Geometry: see drawing. Coordinates: mm, zero at the bounding-box minimum. A direction names the side the tool comes from. Coordinates: 2 decimals unless noted, no trailing zeros. Order: outer loops, then holes, each group sorted by start corner. A loop starts at its lowest first (then second) coordinate and runs counter-clockwise, first axis right, second up. Notation, with made-up numbers: (24.5, -23) - (48.5, -23) arc R9 ccw to (48.5, -10) - close; hole circle Ø6 at (62.25, 18). An arc over 180 degrees is marked (long way). Use a Markdown table: item, result. Add a question column.
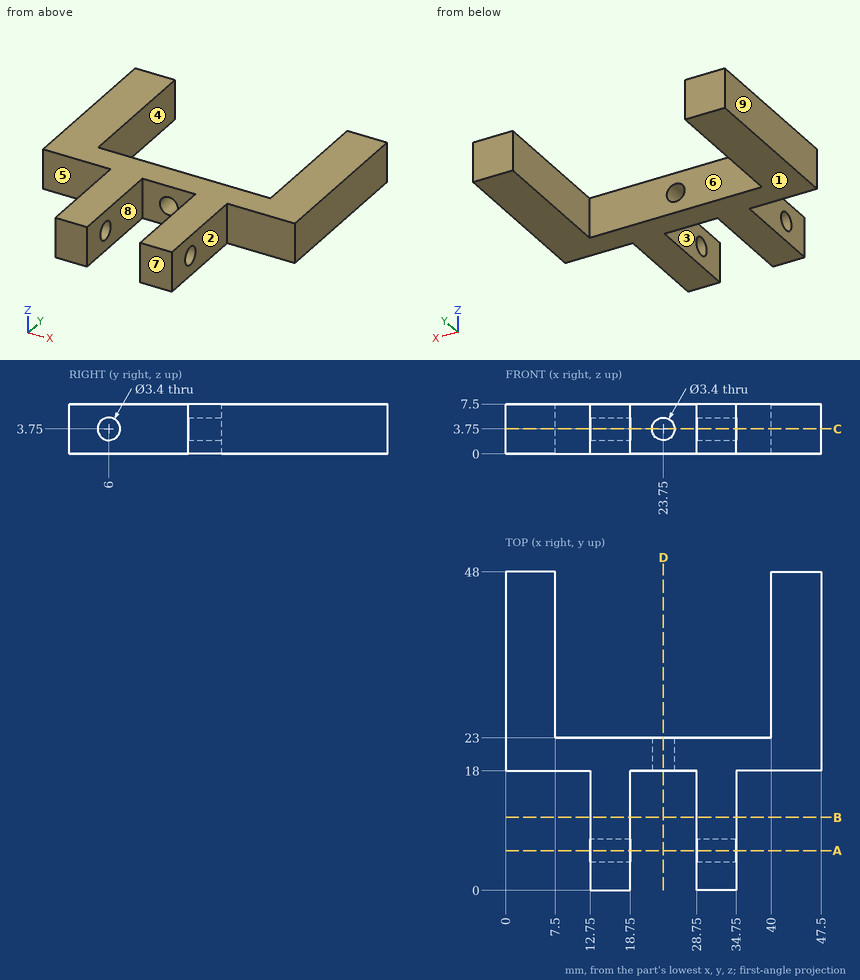
1) Section query B-B (y = 11). Return the cut outline in (x, z), and give its area (3 significant figures).
2) First-contact query: pin 1 (2 mm diameter, centred on y = 10, z = 2, fed in from +X); pin 2 (3 mm diameter, centred on x = 24.5, z = 5, fed in from -Y); pin 3 (1 mm diameter, centred on x = 25.5, z = 2, fed in from +Y); pin 4 (5 mm diameter, centred on x = 25, y = 27, fed in from -Z). Flat tips, straight axial feed; report the tip coordinate or a pass-through.
3) Line query: line 1 (X direction, y = 26, z = 4.5); line 2 (Z direction, x = 31.55, y = 6); line 3 (X direction, y = 14, z = 4.5). Output: solid intervals per line, ascending. Write a range as from..to.
4) Section query C-C (z = 3.75). Return the cut outline in (x, y).
5) Draft query along X for the marked faces 6, 7, 8 and 9. Return one class per face: released by +X, released by -X, zero draft, split by the parting line, or undercut.
6) Section query A-A (y = 6). Return the cut outline in (x, z).
7) Section query D-D (x = 23.75). Return the cut outline in (y, z), and give its area (3 significant figures).
8) Access query for the marked faces 1, 2, 3, 4 and 5. Directions: +Z, -Z, +X, -X, +Y, -Y. A direction counts if a zero-diameter tool reaches every point of the face in a straight line with its end or side. Return the directions, or none.
From the geometry:
| question | item | result |
|---|---|---|
| 1 | outline | (12.75, 0) - (18.75, 0) - (18.75, 7.5) - (12.75, 7.5) - close; (28.75, 0) - (34.75, 0) - (34.75, 7.5) - (28.75, 7.5) - close |
| 1 | area | 90.0 mm^2 |
| 2 | pin 1 | stops at x = 34.75 |
| 2 | pin 2 | stops at y = 18 |
| 2 | pin 3 | stops at y = 23 |
| 2 | pin 4 | passes through |
| 3 | line 1 | x = 0..7.5, 40..47.5 |
| 3 | line 2 | z = 0..2.05, 5.45..7.5 |
| 3 | line 3 | x = 12.75..18.75, 28.75..34.75 |
| 4 | outline | (0, 18) - (12.75, 18) - (12.75, 7.7) - (18.75, 7.7) - (18.75, 18) - (22.05, 18) - (22.05, 23) - (7.5, 23) - (7.5, 48) - (0, 48) - close; (12.75, 0) - (18.75, 0) - (18.75, 4.3) - (12.75, 4.3) - close; (25.45, 18) - (28.75, 18) - (28.75, 7.7) - (34.75, 7.7) - (34.75, 18) - (47.5, 18) - (47.5, 48) - (40, 48) - (40, 23) - (25.45, 23) - close; (28.75, 0) - (34.75, 0) - (34.75, 4.3) - (28.75, 4.3) - close |
| 5 | face 6 | undercut |
| 5 | face 7 | zero draft |
| 5 | face 8 | undercut |
| 5 | face 9 | released by -X |
| 6 | outline | (12.75, 0) - (18.75, 0) - (18.75, 2.05) - (12.75, 2.05) - close; (12.75, 5.45) - (18.75, 5.45) - (18.75, 7.5) - (12.75, 7.5) - close; (28.75, 0) - (34.75, 0) - (34.75, 2.05) - (28.75, 2.05) - close; (28.75, 5.45) - (34.75, 5.45) - (34.75, 7.5) - (28.75, 7.5) - close |
| 7 | outline | (18, 0) - (23, 0) - (23, 2.05) - (18, 2.05) - close; (18, 5.45) - (23, 5.45) - (23, 7.5) - (18, 7.5) - close |
| 7 | area | 20.5 mm^2 |
| 8 | face 1 | -Z, +X, -X, +Y, -Y |
| 8 | face 2 | +Z, -Z, +X, -Y |
| 8 | face 3 | +Z, -Z, -Y |
| 8 | face 4 | +Z, -Z, +Y |
| 8 | face 5 | +Z, -Z, -X, -Y |
